```python
from build123d import *

# Parameters (mm, degrees)
SKETCH_1_R      = 37.5
SKETCH_1_R_2    = 5.05
SKETCH_1_R_3    = 2.05
SKETCH_1_W      = 8.1
SKETCH_1_H      = 2.1
EXTRUDE_1_DEPTH = 2


with BuildPart() as part:
    # 草图1 → 凸台-拉伸1 (new body)
    with BuildSketch(Plane.XY):
        Circle(SKETCH_1_R)
        Circle(SKETCH_1_R_2, mode=Mode.SUBTRACT)
        with Locations((-17.67766953, -17.67766953)):
            Circle(SKETCH_1_R_3, mode=Mode.SUBTRACT)
        with Locations((-17.67766953, 17.67766953)):
            Circle(SKETCH_1_R_3, mode=Mode.SUBTRACT)
        with Locations((17.67766953, 17.67766953)):
            Circle(SKETCH_1_R_3, mode=Mode.SUBTRACT)
        with Locations((17.67766953, -17.67766953)):
            Circle(SKETCH_1_R_3, mode=Mode.SUBTRACT)
        with Locations((-31, -10.05)):
            Circle(SKETCH_1_R_3, mode=Mode.SUBTRACT)
        with Locations(Location((-31, 10.05, 0), (0, 0, 180))):
            Circle(SKETCH_1_R_3, mode=Mode.SUBTRACT)
        with Locations((31, 10.05)):
            Circle(SKETCH_1_R_3, mode=Mode.SUBTRACT)
        with Locations(Location((31, -10.05, 0), (0, 0, 180))):
            Circle(SKETCH_1_R_3, mode=Mode.SUBTRACT)
        with Locations((14.05, 0)):
            Circle(SKETCH_1_R_3, mode=Mode.SUBTRACT)
        with Locations((-14.05, 0)):
            Circle(SKETCH_1_R_3, mode=Mode.SUBTRACT)
        with Locations((0, -33.5)):
            Circle(SKETCH_1_R_3, mode=Mode.SUBTRACT)
        with Locations((16, -10.05)):
            Rectangle(SKETCH_1_W, SKETCH_1_H, mode=Mode.SUBTRACT)
        with Locations((16, 10.05)):
            Rectangle(SKETCH_1_W, SKETCH_1_H, mode=Mode.SUBTRACT)
        with Locations((-16, 10.05)):
            Rectangle(SKETCH_1_W, SKETCH_1_H, mode=Mode.SUBTRACT)
        with Locations((-16, -10.05)):
            Rectangle(SKETCH_1_W, SKETCH_1_H, mode=Mode.SUBTRACT)
    extrude(amount=EXTRUDE_1_DEPTH)


solid = part.part
```
Here's how the part is built. I have some questions about the finished solid (model axes, mm). Coordinates: 2 decimals unless noted, no trailing zeros. Write each loop counter-clockwise with the first axis right and the second up, starting at its lowest first coordinate (ties: lowest second). Pieces come first, ordered by that corner, then holes. Notation, with made-up numbers: (62, 56) -> (112, 56) arc R20 ccw to (112, 92) -> close; hole circle Ø10 at (-11.5, 2.5). An arc over 180 degrees is marked (long way). Use a Markdown table: item, result. Add a question column.
(1) I'm going to push flat-ended pins straight in: P1, Ø5.5, axis at x = 17.68, y = 17.68, coming from the -Z side; P2, Ø1, axis at x = -15.5, z = 1, coming from the +Y side; P3, Ø3.5, axis at x = -14.05, y = 0, coming from the +Z side; P4, Ø0.6, axis at x = 16.5, z = 0.5, coming from the +Y side. Where does each tip first touch, or does it pass through?
(2) We'd pull the mould along X, two halves only. Please class faces 1 (the flat face through (8, 1, 0)), 2 (the cylindrical face through (-32.627, -11.297, 0.986)): +X half, -X half, draft (parallel to the pull), parting line (faces both ways), or undercut.
(3) If we section it at A-A, the plane y = 0: Write out the boundary of the cut face in (x, z), and give its area (3 significant figures).
(4) If we section it at B-B, the plane x = 0: Write out the boundary of the cut face in (y, z).
(5) If we section it at D-D, the plane x = -14.05: Write out the boundary of the cut face in (y, z).
(6) Please list where these lines run through material, in increasing order: line 1 (Y direction, x = 0, z = 1.3); line 2 (X direction, y = 17.5, z = 0.1); line 3 (X direction, y = -19.5, z = 1.05).
(7) If we section it at C-C, the plane z = 0.65: State how many separate pieces and enclosed holes the cut face has, and give its area (3 significant figures).
Outcome:
| question | item | result |
|---|---|---|
| 1 | P1 | stops at z = 0 |
| 1 | P2 | stops at y = 34.37 |
| 1 | P3 | passes through |
| 1 | P4 | stops at y = 33.82 |
| 2 | face 1 | draft |
| 2 | face 2 | undercut |
| 3 | outline | (-37.5, 0) -> (-16.1, 0) -> (-16.1, 2) -> (-37.5, 2) -> close; (-12, 0) -> (-5.05, 0) -> (-5.05, 2) -> (-12, 2) -> close; (5.05, 0) -> (12, 0) -> (12, 2) -> (5.05, 2) -> close; (16.1, 0) -> (37.5, 0) -> (37.5, 2) -> (16.1, 2) -> close |
| 3 | area | 113 mm^2 |
| 4 | outline | (-37.5, 0) -> (-35.55, 0) -> (-35.55, 2) -> (-37.5, 2) -> close; (-31.45, 0) -> (-5.05, 0) -> (-5.05, 2) -> (-31.45, 2) -> close; (5.05, 0) -> (37.5, 0) -> (37.5, 2) -> (5.05, 2) -> close |
| 5 | outline | (-34.77, 0) -> (-11.1, 0) -> (-11.1, 2) -> (-34.77, 2) -> close; (-9, 0) -> (-2.05, 0) -> (-2.05, 2) -> (-9, 2) -> close; (2.05, 0) -> (9, 0) -> (9, 2) -> (2.05, 2) -> close; (11.1, 0) -> (34.77, 0) -> (34.77, 2) -> (11.1, 2) -> close |
| 6 | line 1 | y = -37.5 to -35.55, -31.45 to -5.05, 5.05 to 37.5 |
| 6 | line 2 | x = -33.17 to -19.72, -15.64 to 15.64, 19.72 to 33.17 |
| 6 | line 3 | x = -32.03 to -18.62, -16.74 to 16.74, 18.62 to 32.03 |
| 7 | separate pieces | 1 |
| 7 | enclosed holes | 16 |
| 7 | area | 4,120 mm^2 |
